Check sheet for the modelled part. Datum: model origin and axes. Units: mm. Face numbers are marked on the shaded views. Coordinates: 2 decimals unless noted, no trailing zeros. Loops run counter-clockwise (first coordinate to the right, second up) from the corner with the lowest first, then second, coordinate; pieces in that order, holes last.
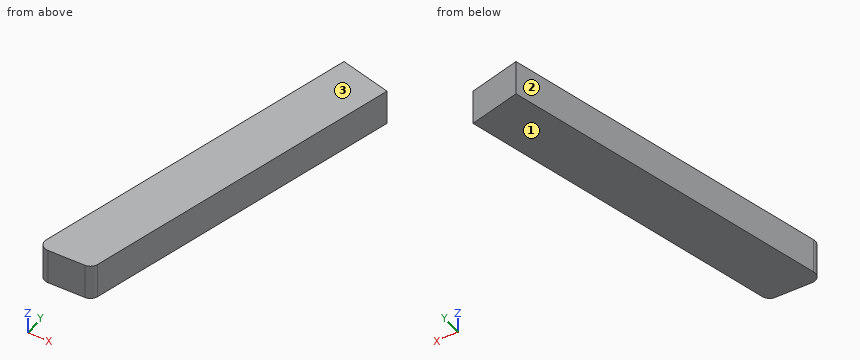
```python
from build123d import *

# Parameters (mm, degrees)
BOSS_EXTRU_1_DEPTH = 20
CONG_1_R           = 5


with BuildPart() as part:
    # Esquisse1 → Boss.-Extru.1 (new body)
    with BuildSketch(Plane.XY):
        Polygon((0, 0), (31.058285412, 0), (80.741583809, 185.420593905), (51.763809021, 193.185165258), align=None)
    extrude(amount=BOSS_EXTRU_1_DEPTH)

    # Congé1
    cong_1_edges = [part.edges().sort_by_distance(p)[0] for p in [
        (31.058285412, 0, 10),
        (0, 0, 10),
    ]]
    fillet(cong_1_edges, radius=CONG_1_R)


solid = part.part
```
1) Section check B-B on y = 73. Enter the section's corners in (x, z), plus the area to 3 significant figures.
Answer sheet:
outline: (19.56, 0) - (50.62, 0) - (50.62, 20) - (19.56, 20) - close
area: 621 mm2
2) Scan lines: line 1 (X direction, y = 116, z = 12.25); line 2 (X direction, y = 16.5, z = 3.25). Record each from-to range of solid material in increasing order.
Answer sheet:
line 1: x = 31.08 to 62.14
line 2: x = 4.42 to 35.48
3) Section check A-A on z = 1.75. Enter the section's corners in (x, y), plus the area to 3 significant figures.
Answer sheet:
outline: (1.69, 6.29) arc R5 ccw to (6.52, 0) - (27.22, 0) arc R5 ccw to (32.05, 3.71) - (80.74, 185.42) - (51.76, 193.19) - close
area: 5,870 mm2
4) Depth check by flat-ended pin: pin 1 (1 mm diameter, centred on y = 98.5, z = 2.5, fed in from +X); pin 2 (4 mm diameter, centred on y = 27.5, z = 5.5, fed in from -X); pin 3 (5 mm diameter, centred on y = 61, z = 2.5, fed in from +X). Enter the tip coordinate at first touch or a pass-through.
Answer sheet:
pin 1: stops at x = 57.59
pin 2: stops at x = 6.83
pin 3: stops at x = 48.07
5) Mould release check, pull along Z, two halves, no side actions. Record for the marked faces 1, 2 and 3: +Z half, -Z half, draft (parallel to the pull), parting line (faces both ways), or undercut.
Answer sheet:
face 1: -Z half
face 2: draft
face 3: +Z half
6) Section check C-C on x = 12. Enter the section's corners in (y, z), plus the area to 3 significant figures.
Answer sheet:
outline: (0, 0) - (44.78, 0) - (44.78, 20) - (0, 20) - close
area: 896 mm2
